Here's the drawing with two shaded views (mm, measured from the low corner). I have some questions. A direction names the side the tool comes from. Coordinates: 2 decimals unless noted, no trailing zeros. Loops run counter-clockwise (first coordinate to the right, second up) from the corner with the lowest first, then second, coordinate; pieces in that order, holes last. Notation, with made-up numbers: (-0.75, 48.5) -> (46.25, 48.5) arc R11 ccw to (46.25, 69.5) -> close; hole circle Ø9 at (55, -6.75). An arc over 180 degrees is marked (long way). Answer as a JSON object with one key per item and string values. Group by question number.
Q1. I need wall thicknesses on line 1 (Z direction, x = 7.5, y = 29); line 2 (Y direction, x = 2.25, z = 7); line 3 (Z direction, x = 10.5, y = 19) (1 decimal). Which ranges of each line are inside material? Lowest first, please.
Q2. I want a section at A-A on x = 4. Write out the boundary of the cut face in (y, z).
Q3. I'm going to push flat-ended pins straight in: pin 1 (6.5 mm diameter, centred on x = 6.5, y = 32.5, fed in from +Z); pin 2 (6 mm diameter, centred on x = 9.5, z = 22, fed in from -Y); pin 3 (3 mm diameter, centred on x = 3, z = 12.5, fed in from +Y). Where does each tip first touch, or does it pass through?
Q4. I want a section at B-B on z = 28. Write out the boundary of the cut face in (x, y).
Q5. I want a section at C-C on y = 32. Write out the boundary of the cut face in (x, z), then the cut area to 3 significant figures.
Q6. On a 3-axis mill with a long thin cutter (end or side, diameter ignored), from which of +Z, -Z, +X, -X, +Y, -Y can I reach the whole of each face in a straight line? I mean the marked faces 1, 2 and 3. Say none if no direction works.
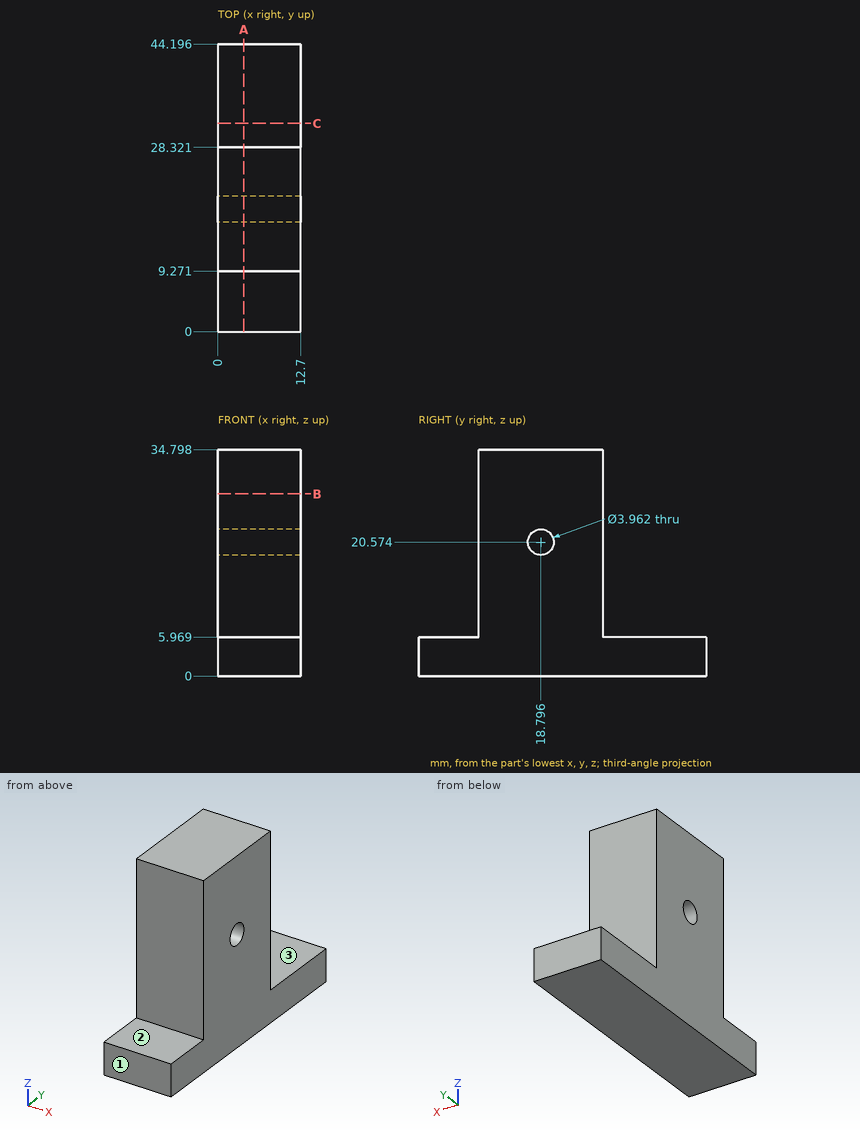
Result set:
{
 "1": {"line 1": "z = 0 to 5.97", "line 2": "y = 9.27 to 28.32", "line 3": "z = 0 to 18.6, 22.5 to 34.8"},
 "2": {"outline": "(0, 0) -> (44.2, 0) -> (44.2, 5.97) -> (28.32, 5.97) -> (28.32, 34.8) -> (9.27, 34.8) -> (9.27, 5.97) -> (0, 5.97) -> close; hole circle Ø3.96 at (18.8, 20.57)"},
 "3": {"pin 1": "stops at z = 5.97", "pin 2": "stops at y = 9.27", "pin 3": "stops at y = 28.32"},
 "4": {"outline": "(0, 9.27) -> (12.7, 9.27) -> (12.7, 28.32) -> (0, 28.32) -> close"},
 "5": {"outline": "(0, 0) -> (12.7, 0) -> (12.7, 5.97) -> (0, 5.97) -> close", "area": "75.8 mm²"},
 "6": {"face 1": "+Z, -Z, +X, -X, -Y", "face 2": "+Z, +X, -X, -Y", "face 3": "+Z, +X, -X, +Y"}
}
